```python
from build123d import *


with BuildPart() as part:
    # Sketch1 → Rivoluzione1 (revolve)
    with BuildSketch(Plane.XY):
        with BuildLine():
            Line((-13, 252.3), (-18.085, 252.3))
            Line((-18.085, 252.3), (-19.1, 227.3))
            Line((-19.1, 227.3), (-31.5, 227.3))
            Line((-31.5, 227.3), (-31.5, 212.3))
            Line((-31.5, 212.3), (-27.5, 210.8))
            Line((-27.5, 210.8), (-27.5, 206.8))
            Line((-27.5, 206.8), (-31.5, 205.3))
            Line((-31.5, 205.3), (-31.5, 200.3))
            Line((-31.5, 200.3), (-20, 200.3))
            Line((-20, 200.3), (-19.75, 200.3))
            ThreePointArc((-19.75, 200.3), (-19.926776695, 200.226776695), (-20, 200.05))
            Line((-20, 200.05), (-20, 2.444337567))
            ThreePointArc((-20, 2.444337567), (-19.966506351, 2.319337567), (-19.875, 2.227831216))
            Line((-19.875, 2.227831216), (-15.669872981, -0.2))
            Line((-15.669872981, -0.2), (-13.5, -0.2))
            Line((-13.5, -0.2), (-13.5, 0))
            Line((-13.5, 0), (-2.5, 0))
            Line((-2.5, 0), (-2.5, 15))
            Line((-2.5, 15), (0, 15))
            Line((0, 15), (0, 218.3))
            Line((0, 218.3), (-13, 218.3))
            Line((-13, 218.3), (-13, 223.3))
            Line((-13, 223.3), (-14, 223.3))
            ThreePointArc((-14, 223.3), (-15.414213562, 223.885786438), (-16, 225.3))
            Line((-16, 225.3), (-16, 243.3))
            ThreePointArc((-16, 243.3), (-15.414213562, 244.714213562), (-14, 245.3))
            Line((-14, 245.3), (-13, 245.3))
            Line((-13, 245.3), (-13, 252.3))
        make_face()
    revolve(axis=Axis((0, 0, 0), (0, 1, 0)))


with BuildPart() as part_1:
    # Corpo-Sposta/copia1: moved
    add(part.part.moved(Location((0, -209, 0))))


solid = part_1.part
```
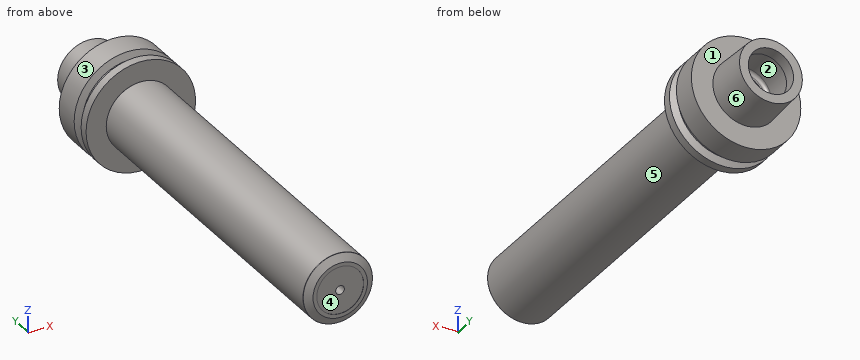
Could you check a few things on this model? Use its own coordinates, in mm. Face numbers are marked on the shaded views. A direction names the side the tool comes from. Coordinates: 2 decimals unless noted, no trailing zeros. Order: outer loops, then holes, each group sorted by start corner. A loop starts at its lowest first (then second) coordinate and runs counter-clockwise, first axis right, second up. Notation, with made-up numbers: M 40,58 L 73,58 A10 ccw 73,73 Z; hole C 64.25,-34.75 d11. An arc over 180 degrees is marked long. Use a Markdown table: item, result. Add a question column.
Q1. I'm going to push flat-ended pins straight in: pin 1 (12 mm diameter, centred on x = -5.5, y = -94, fed in from -Z); pin 2 (2.5 mm diameter, centred on x = 1, z = 1, fed in from -Y); pin 3 (3 mm diameter, centred on y = -87, z = -11.5, fed in from +X). Where does each tip first touch, or does it pass through?
Q2. If I drill on L1, parallel to Y at x = -7, z = 3.5; L2, parallel to Z at x = 0, y = 39; L3, parallel to Z at x = 0, y = 12.8, over which ranges is the centre line in solid material (lowest first)?
Q3. I want a section at A-A on y = -173. List the corners of the cut face in (x, z) for me, then the cut area to 3 significant figures.
Q4. Which directions (+Z, -Z, +X, -X, +Y, -Y) give clear straight access to the entire face, cutting with the end or side of a thin tool? Please do the marked faces 5 and 6.
Q5. We'd pull the mould along Z, two halves only. Please class the marked faces 1, 2, 3 and 4: pulls with the +Z half, pulls with the -Z half, needs draft (parallel to the pull), parting line crosses it, or undercut.
Checked values:
| question | item | result |
|---|---|---|
| 1 | pin 1 | z = -20 |
| 1 | pin 2 | y = -209 |
| 1 | pin 3 | x = 17.32 |
| 2 | L1 | -209 to 9.3 |
| 2 | L2 | -18.26 to -13, 13 to 18.26 |
| 2 | L3 | -31.5 to -13, 13 to 31.5 |
| 3 | outline | C 0,0 d40 |
| 3 | area | 1,260 mm² |
| 4 | face 5 | -Y |
| 4 | face 6 | +Y |
| 5 | face 1 | needs draft |
| 5 | face 2 | undercut |
| 5 | face 3 | parting line crosses it |
| 5 | face 4 | undercut |
